Work out the finished part from the listing and answer in its coordinate system (mm). Give positions to 0.01 mm unless a question says otherwise; leave off trailing zeros. Write each loop counter-clockwise with the first axis right and the second up, starting at its lowest first coordinate (ties: lowest second). Pieces come first, ordered by that corner, then holes. Notation, with made-up numbers: (54.25, 72.25) -> (65.25, 72.25) arc R7 ccw to (65.25, 80.25) -> close; hole circle Ø11 at (32, -14.75). An arc over 180 degrees is marked (long way). Use a Markdown table: item, result. Add a question column.
Q1. Section C-C, the plane y = -472 is taken. Give the vertices of the cut face in (x, z).
Q2. Section B-B, the plane z = -337 is taken. Give the vertices of the cut face in (x, y), plus the area to 3 significant figures.
Q3. This flat-tipped pin is pushed along its axis until it touches: pin 1 Ø5 at (x, y) = (-14, -482.5) entering from -Z. Where does it stop, or does it pass through?
Q4. Consider line 1 (Z direction, x = -42.5, y = -516); line 2 (Y direction, x = -99, z = -338). Determine where each line is inside the solid, lowest interval first.
Q5. Section A-A, the plane x = 87 is taken. Give the vertices of the cut face in (y, z).
from build123d import *

# Parameters (mm, degrees)
F0_W     = 377.825
F0_H     = 860.425
F1_DEPTH = 514.35
F2_DEPTH = 25.4
F3_W     = 69.85
F3_H     = 107.95
F4_DEPTH = 403.226
F5_W     = 403.225
F5_H     = 752.475
F6_DEPTH = 44.45


with BuildPart() as f1:
    # F0 (on Front) → F1 (new body)
    with BuildSketch(Plane.XZ):
        Rectangle(F0_W, F0_H)
    extrude(amount=F1_DEPTH)

    # F2 (add): a face of the model
    f2_faces = [f1.faces().sort_by_distance(p)[0] for p in [
        (188.9125, -257.175, 0),
    ]]
    extrude(f2_faces, amount=F2_DEPTH)

    # F3 (on face) → F4 (cut, through all)
    with BuildSketch(Plane.YZ.offset(214.3125)):
        with Locations((-479.425, -376.2375)):
            Rectangle(F3_W, F3_H)
    extrude(amount=-F4_DEPTH, mode=Mode.SUBTRACT)

    # F5 (on face) → F6 (join)
    with BuildSketch(Plane.XZ.offset(514.35)):
        with Locations((12.7, 53.975)):
            Rectangle(F5_W, F5_H)
    extrude(amount=F6_DEPTH)


solid = f1.part
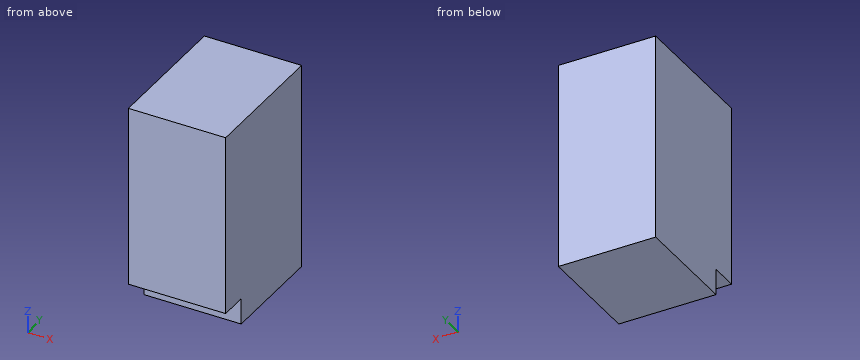
Result set:
| question | item | result |
|---|---|---|
| 1 | outline | (-188.91, -322.26) -> (214.31, -322.26) -> (214.31, 430.21) -> (-188.91, 430.21) -> close |
| 2 | outline | (-188.91, -444.5) -> (214.31, -444.5) -> (214.31, 0) -> (-188.91, 0) -> close |
| 2 | area | 179,000 mm2 |
| 3 | pin 1 | stops at z = -322.26 |
| 4 | line 1 | z = -322.26 to 430.21 |
| 4 | line 2 | y = -444.5 to 0 |
| 5 | outline | (-558.8, -322.26) -> (-444.5, -322.26) -> (-444.5, -430.21) -> (0, -430.21) -> (0, 430.21) -> (-558.8, 430.21) -> close |
